Input: part model. Units: mm. Frame: model coordinates. Face numbers are marked on the shaded views. Give positions to 0.01 mm unless a question says otherwise; leave off trailing zeros. Loops run counter-clockwise (first coordinate to the right, second up) from the corner with the lowest first, then second, coordinate; pieces in that order, holes last. Notation, with made-up numbers: (30.5, 1.25) - (81.5, 1.25) arc R23 cw to (81.5, 26.25) - close; hole circle Ø9 at (15, 50.5). An arc over 180 degrees is marked (long way). Answer as a JSON object with one key per item and string values.
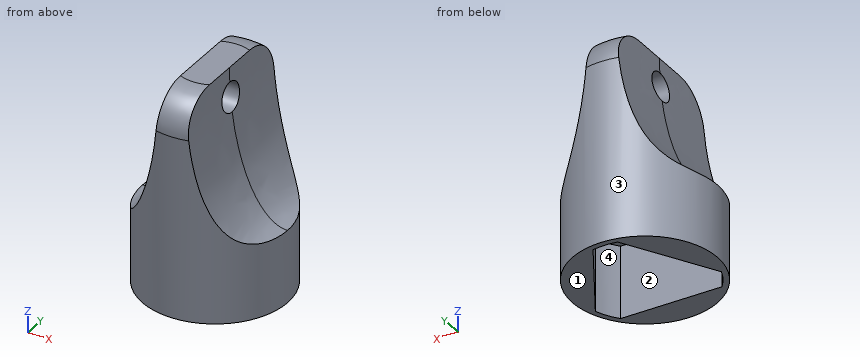
from build123d import *

# Parameters (mm, degrees)
F2_R     = 10
F3_DEPTH = 10
F4_DEPTH = 20
F6_DEPTH = 12.5
F7_R     = 2
F8_DEPTH = 12.5
F9_R     = 5


with BuildPart() as f3:
    # F2 (on Top) → F3 (new body)
    with BuildSketch(Plane.XY):
        Circle(F2_R)
        with BuildLine():
            ThreePointArc((7, -6), (0, -9.2195444573), (-7, -6))
            ThreePointArc((-7, -6), (-7.9843597113, -4.6097722286), (-8.6961524227, -3.0621778265))
            ThreePointArc((-8.6961524227, -3.0621778265), (-7.9843597113, 4.6097722286), (-1.6961524227, 9.0621778265))
            ThreePointArc((-1.6961524227, 9.0621778265), (0, 9.2195444573), (1.6961524227, 9.0621778265))
            ThreePointArc((1.6961524227, 9.0621778265), (7.0935799378, 5.8890681492), (9.2195444573, 0))
            ThreePointArc((9.2195444573, 0), (9.0877545045, -1.553292653), (8.6961524227, -3.0621778265))
            ThreePointArc((8.6961524227, -3.0621778265), (7.9843597113, -4.6097722286), (7, -6))
        make_face(mode=Mode.SUBTRACT)
        with BuildLine():
            Line((-8.6961524227, -3.0621778265), (-5.1961524227, 3))
            Line((-5.1961524227, 3), (-1.6961524227, 9.0621778265))
            ThreePointArc((-1.6961524227, 9.0621778265), (-7.9843597113, 4.6097722286), (-8.6961524227, -3.0621778265))
        make_face()
        with BuildLine():
            Line((7, -6), (0, -6))
            Line((0, -6), (-7, -6))
            ThreePointArc((-7, -6), (0, -9.2195444573), (7, -6))
        make_face()
        with BuildLine():
            Line((1.6961524227, 9.0621778265), (5.1961524227, 3))
            Line((5.1961524227, 3), (8.6961524227, -3.0621778265))
            ThreePointArc((8.6961524227, -3.0621778265), (9.0877545045, -1.553292653), (9.2195444573, 0))
            ThreePointArc((9.2195444573, 0), (7.0935799378, 5.8890681492), (1.6961524227, 9.0621778265))
        make_face()
    extrude(amount=-F3_DEPTH)

    # F2 (on Top) → F4 (join)
    with BuildSketch(Plane.XY):
        Circle(F2_R)
        with BuildLine():
            ThreePointArc((7, -6), (0, -9.2195444573), (-7, -6))
            ThreePointArc((-7, -6), (-7.9843597113, -4.6097722286), (-8.6961524227, -3.0621778265))
            ThreePointArc((-8.6961524227, -3.0621778265), (-7.9843597113, 4.6097722286), (-1.6961524227, 9.0621778265))
            ThreePointArc((-1.6961524227, 9.0621778265), (0, 9.2195444573), (1.6961524227, 9.0621778265))
            ThreePointArc((1.6961524227, 9.0621778265), (7.0935799378, 5.8890681492), (9.2195444573, 0))
            ThreePointArc((9.2195444573, 0), (9.0877545045, -1.553292653), (8.6961524227, -3.0621778265))
            ThreePointArc((8.6961524227, -3.0621778265), (7.9843597113, -4.6097722286), (7, -6))
        make_face(mode=Mode.SUBTRACT)
        with BuildLine():
            Line((0, -6), (0, 0))
            Line((0, 0), (-5.1961524227, 3))
            Line((-5.1961524227, 3), (-8.6961524227, -3.0621778265))
            ThreePointArc((-8.6961524227, -3.0621778265), (-7.9843597113, -4.6097722286), (-7, -6))
            Line((-7, -6), (0, -6))
        make_face()
        with BuildLine():
            Line((-8.6961524227, -3.0621778265), (-5.1961524227, 3))
            Line((-5.1961524227, 3), (-1.6961524227, 9.0621778265))
            ThreePointArc((-1.6961524227, 9.0621778265), (-7.9843597113, 4.6097722286), (-8.6961524227, -3.0621778265))
        make_face()
        with BuildLine():
            Line((-5.1961524227, 3), (0, 0))
            Line((0, 0), (5.1961524227, 3))
            Line((5.1961524227, 3), (1.6961524227, 9.0621778265))
            ThreePointArc((1.6961524227, 9.0621778265), (0, 9.2195444573), (-1.6961524227, 9.0621778265))
            Line((-1.6961524227, 9.0621778265), (-5.1961524227, 3))
        make_face()
        with BuildLine():
            Line((5.1961524227, 3), (0, 0))
            Line((0, 0), (0, -6))
            Line((0, -6), (7, -6))
            ThreePointArc((7, -6), (7.9843597113, -4.6097722286), (8.6961524227, -3.0621778265))
            Line((8.6961524227, -3.0621778265), (5.1961524227, 3))
        make_face()
        with BuildLine():
            Line((1.6961524227, 9.0621778265), (5.1961524227, 3))
            Line((5.1961524227, 3), (8.6961524227, -3.0621778265))
            ThreePointArc((8.6961524227, -3.0621778265), (9.0877545045, -1.553292653), (9.2195444573, 0))
            ThreePointArc((9.2195444573, 0), (7.0935799378, 5.8890681492), (1.6961524227, 9.0621778265))
        make_face()
        with BuildLine():
            Line((7, -6), (0, -6))
            Line((0, -6), (-7, -6))
            ThreePointArc((-7, -6), (0, -9.2195444573), (7, -6))
        make_face()
    extrude(amount=F4_DEPTH)

    # F5 (on Front) → F6 (cut, symmetric)
    with BuildSketch(Plane.XZ):
        with BuildLine():
            Line((-10, 0), (-10, 20))
            Line((-10, 20), (-2, 20))
            add(Edge.make_bspline(
                [(-2, 20), (-2, 68.2842712475), (-15.6568542495, 34.1421356237), (-29.313708499, 0), (-10, 0)],
                knots=[4.7123889804, 4.7123889804, 4.7123889804, 7.0685834706, 7.0685834706, 9.4247779608, 9.4247779608, 9.4247779608], degree=2, weights=[1, 0.3826834324, 1, 0.3826834324, 1]))
        make_face()
        with BuildLine():
            Line((-2, 20), (-10, 20))
            Line((-10, 20), (-10, 0))
            add(Edge.make_bspline(
                [(-10, 0), (-2, 0), (-2, 20)],
                knots=[3.1415926536, 3.1415926536, 3.1415926536, 4.7123889804, 4.7123889804, 4.7123889804], degree=2, weights=[1, 0.7071067812, 1]))
        make_face()
        with BuildLine():
            add(Edge.make_bspline(
                [(2, 20), (2, -14.6410161514), (14, 2.6794919243), (26, 20), (14, 37.3205080757), (2, 54.6410161514), (2, 20)],
                knots=[4.7123889804, 4.7123889804, 4.7123889804, 6.8067840828, 6.8067840828, 8.9011791852, 8.9011791852, 10.9955742876, 10.9955742876, 10.9955742876], degree=2, weights=[1, 0.5, 1, 0.5, 1, 0.5, 1]))
        make_face()
    extrude(amount=F6_DEPTH, both=True, mode=Mode.SUBTRACT)

    # F7 (on Right) → F8 (cut, symmetric)
    with BuildSketch(Plane.YZ):
        with Locations((0, 16)):
            Circle(F7_R)
    extrude(amount=F8_DEPTH, both=True, mode=Mode.SUBTRACT)

    # F9
    f9_edges = [f3.edges().sort_by_distance(p)[0] for p in [
        (0, 10, 20),
        (0, -10, 20),
    ]]
    fillet(f9_edges, radius=F9_R)


solid = f3.part
Item 1: Material intervals for line 1 (Z direction, x = 0.55, y = 0); line 2 (Y direction, x = 0.5, z = 16); line 3 (X direction, y = 2.75, z = -7.5), sorted ascending. Write a range as [from, to].
Geometry check:
{"line 1": "z = [0, 14], [18, 20]", "line 2": "y = [-9.89, -2], [2, 9.89]", "line 3": "x = [-9.61, -5.34], [5.34, 9.61]"}
Item 2: Contact query for flat-ended pins moving along their axis: P1, Ø4.5, axis at x = -3.5, y = 0.5, coming from the -Z side; P2, Ø8, axis at y = 2.5, z = 4.5, coming from the -X side; P3, Ø10, axis at y = 3, z = 9, coming from the -X side. Output: stop coordinate, or through.
Geometry check:
{"P1": "stops at z = 0", "P2": "stops at x = -8.22", "P3": "stops at x = -5.2"}
Item 3: Mould query, pull axis X, two halves, no side actions, for the marked faces 1, 2, 3 and 4. Classes: released by +X, released by -X, zero draft, split by the parting line, or undercut.
Geometry check:
{"face 1": "zero draft", "face 2": "undercut", "face 3": "split by the parting line", "face 4": "undercut"}
Item 4: Cut plane A-A (z = -3.5). Return loops of the section in (x, y), then the cut area to 3 significant figures.
Geometry check:
{"outline": "circle Ø20 at (0, 0); hole (-8.7, -3.06) arc R9.22 ccw to (-7, -6) - (7, -6) arc R9.22 ccw to (8.7, -3.06) - (1.7, 9.06) arc R9.22 ccw to (-1.7, 9.06) - close", "area": "141 mm2"}
